from build123d import *

# Parameters (mm, degrees)
SKETCH1_R              = 5
SKETCH1_R_2            = 3.96875
BEARING_COLLAR_DEPTH   = 6.35
SKETCH1_3_R            = 3.96875
CENTER_SPINDLE_DEPTH   = 4.7625
F_10_CLEARANCE_HOLE1_D = 4.9784


with BuildPart() as part:
    # Sketch1 → Bearing Collar (new body)
    # profile 1 of 2: a face of its own
    with BuildSketch(Plane(origin=(0, 0, 0), x_dir=(1, 0, 0), z_dir=(0, 1, 0))):
        with Locations(Location((0, 0, 0), (0, 0, 270))):
            Circle(SKETCH1_R)
        Circle(SKETCH1_R_2, mode=Mode.SUBTRACT)
    # profile 2 of 2: a face of its own
    with BuildSketch(Plane(origin=(0, 0, 0), x_dir=(1, 0, 0), z_dir=(0, 1, 0))):
        Circle(SKETCH1_R_2)
    extrude(amount=BEARING_COLLAR_DEPTH)

    # Sketch1_3 → Center Spindle (add)
    with BuildSketch(Plane(origin=(0, 0, 0), x_dir=(1, 0, 0), z_dir=(0, 1, 0))):
        with Locations(Location((0, 0, 0), (0, 0, 270))):
            Circle(SKETCH1_3_R)
    extrude(amount=-CENTER_SPINDLE_DEPTH)

    # 10 Clearance Hole1 (through all)
    with Locations(Plane(origin=(0, -4.7625, 0), x_dir=(0, 0, -1), z_dir=(0, -1, 0))):
        with Locations((0, 0)):
            Hole(F_10_CLEARANCE_HOLE1_D / 2)


solid = part.part
Source: CAD feature listing. Evaluate the final solid. Frame: model axes, mm. A direction names the side the tool comes from. Give positions to 0.01 mm unless a question says otherwise; leave off trailing zeros. Write each loop counter-clockwise with the first axis right and the second up, starting at its lowest first coordinate (ties: lowest second). Pieces come first, ordered by that corner, then holes. Notation, with made-up numbers: (8.25, 35.5) -> (65.25, 35.5) arc R8 cw to (65.25, 45.5) -> close; hole circle Ø3 at (-26, 83.25). An arc over 180 degrees is marked (long way). Write item = value, one per line.
Q1. Cut plane B-B on z = 0. Return loops of the section in (x, y), then the cut area to 3 significant figures.
Here are the results:
outline = (-5, 0) -> (-3.97, 0) -> (-3.97, -4.76) -> (-2.49, -4.76) -> (-2.49, 6.35) -> (-5, 6.35) -> close; (2.49, -4.76) -> (3.97, -4.76) -> (3.97, 0) -> (5, 0) -> (5, 6.35) -> (2.49, 6.35) -> close
area = 46.0 mm²
Q2. Reachability of faces 4 (the face through (-3, 0, -3)), 5 (the face through (-4.88, 3.13, -1.08)) from +Z, -Z, +X, -X, +Y, -Y: full face, straight path, thin tool, end or side. Return the list, or none.
Here are the results:
face_4 = -Y
face_5 = +Y, -Y
Q3. First-contact query: pin 1 (1.5 mm diameter, centred on x = 1, y = 1.5, fed in from +Z); pin 2 (4 mm diameter, centred on x = 0, z = 0, fed in from -Y). Flat tips, straight axial feed; report the tip coordinate or a pass-through.
Here are the results:
pin_1 = 4.99
pin_2 = through
Q4. Line query: line 1 (X direction, y = 2.25, z = 0); line 2 (X direction, y = -1, z = 0); line 3 (Y direction, x = -0.5, z = -4). Output: solid intervals per line, ascending. Write a range as from..to.
Here are the results:
line_1 = -5..-2.49, 2.49..5
line_2 = -3.97..-2.49, 2.49..3.97
line_3 = 0..6.35
Q5. Mould query, pull axis Z, two halves, no side actions, for faces 1 (the face through (0.748, 0.872, 2.374)), 2 (the face through (-3.874, -2.348, -0.86)), 3 (the face through (-2, 6.35, 2)). Classes: +Z half, -Z half, draft (parallel to the pull), parting line (faces both ways), or undercut.
Here are the results:
face_1 = undercut
face_2 = parting line
face_3 = draft
Q6. Cut plane C-C on y = 3.25. Return loops of the section in (x, z).
Here are the results:
outline = circle Ø10 at (0, 0); hole circle Ø4.98 at (0, 0)
Q7. Cut plane A-A on x = 0. Return loops of the section in (y, z), then the cut area to 3 significant figures.
Here are the results:
outline = (-4.76, -3.97) -> (0, -3.97) -> (0, -5) -> (6.35, -5) -> (6.35, -2.49) -> (-4.76, -2.49) -> close; (-4.76, 2.49) -> (6.35, 2.49) -> (6.35, 5) -> (0, 5) -> (0, 3.97) -> (-4.76, 3.97) -> close
area = 46.0 mm²
Q8. Cut plane D-D on x = 3.25. Return loops of the section in (y, z).
Here are the results:
outline = (-4.76, -2.28) -> (0, -2.28) -> (0, -3.8) -> (6.35, -3.8) -> (6.35, 3.8) -> (0, 3.8) -> (0, 2.28) -> (-4.76, 2.28) -> close
